from build123d import *

# Parameters (mm, degrees)
F2_R     = 1.575
F3_DEPTH = 4
F4_COUNT = 2
F5_R     = 5
F6_R     = 2.5
F7_R     = 0.5
F8_SIZE  = 1
F9_SIZE  = 0.25


with BuildPart() as f1:
    # F0 (on Right) → F1 (revolve)
    with BuildSketch(Plane.YZ):
        with BuildLine():
            Line((16.36, 0), (14, 0))
            Line((14, 0), (14, -4))
            Line((14, -4), (18, -4))
            Line((18, -4), (18, -1.64))
            ThreePointArc((18, -1.64), (16.8403448789, -1.1596551211), (16.36, 0))
        make_face()
    revolve(axis=Axis((0, 0, -0.7442336064), (0, 0, -1)))

    # F2 (on face) → F3 (join, through all)
    with BuildSketch(Plane.XY):
        with BuildLine():
            Line((-8.1, 2.5), (-9.9233440343, 2.5))
            ThreePointArc((-9.9233440343, 2.5), (-10.7587622743, 3.003635948), (-11.7060032895, 3.2366751357))
            ThreePointArc((-11.7060032895, 3.2366751357), (-12.8521864455, 3.9515520359), (-12.95875, 5.2981882222))
            ThreePointArc((-12.95875, 5.2981882222), (-14, 0), (-12.95875, -5.2981882222))
            ThreePointArc((-12.95875, -5.2981882222), (-12.8521864455, -3.9515520359), (-11.7060032895, -3.2366751357))
            ThreePointArc((-11.7060032895, -3.2366751357), (-10.7587622743, -3.003635948), (-9.9233440343, -2.5))
            Line((-9.9233440343, -2.5), (-8.1, -2.5))
            Line((-8.1, -2.5), (-8.1, -5))
            Line((-8.1, -5), (-6.6, -5))
            Line((-6.6, -5), (-4.1, -2.5))
            Line((-4.1, -2.5), (-4.1, 2.5))
            Line((-4.1, 2.5), (-6.6, 5))
            Line((-6.6, 5), (-8.1, 5))
            Line((-8.1, 5), (-8.1, 2.5))
        make_face()
        with Locations((-12, 0)):
            Circle(F2_R, mode=Mode.SUBTRACT)
    extrude(amount=-F3_DEPTH)

    # F4: F1 ×2 about axis
    f4_axis = Axis((0, 0, 0), (0, 0, -1))


with BuildPart() as f1_1:
    add(f1.part)
    for i in range(1, F4_COUNT):
        add(f1.part.rotate(f4_axis, i * 360 / F4_COUNT))

    # F5
    f5_edges = [f1_1.edges().sort_by_distance(p)[0] for p in [
        (-4.1, -2.5, -2),
        (-4.1, 2.5, -2),
        (4.1, 2.5, -2),
        (4.1, -2.5, -2),
    ]]
    fillet(f5_edges, radius=F5_R)

    # F6
    f6_edges = [f1_1.edges().sort_by_distance(p)[0] for p in [
        (-9.923344, 2.5, -2),
        (-9.923344, -2.5, -2),
        (9.923344, 2.5, -2),
        (9.923344, -2.5, -2),
    ]]
    fillet(f6_edges, radius=F6_R)

    # F7
    f7_edges = [f1_1.edges().sort_by_distance(p)[0] for p in [
        (-8.1, 2.5, -2),
        (-8.1, -2.5, -2),
        (8.1, -2.5, -2),
        (8.1, 2.5, -2),
    ]]
    fillet(f7_edges, radius=F7_R)

    # F8
    f8_edges = [f1_1.edges().sort_by_distance(p)[0] for p in [
        (0, -18, -4),
    ]]
    chamfer(f8_edges, length=F8_SIZE)

    # F9
    f9_edges = [f1_1.edges().sort_by_distance(p)[0] for p in [
        (13.575, 0, -4),
        (-13.575, 0, -4),
    ]]
    chamfer(f9_edges, length=F9_SIZE)


solid = f1_1.part
Check sheet for the modelled part. Datum: model origin and axes. Units: mm. Give positions to 0.01 mm unless a question says otherwise; leave off trailing zeros. Order: outer loops, then holes, each group sorted by start corner. A loop starts at its lowest first (then second) coordinate and runs counter-clockwise, first axis right, second up. Notation, with made-up numbers: M 59,-13 L 71,-13 A15 cw 71,8 Z; hole C -9.5,-17 d4. An arc over 180 degrees is marked long. Answer as CSV lines item,"result". Start each with the question number.
Item 1: Cross-section at A-A on x = 0. Enter the section's corners in (y, z), plus the area to 3 significant figures.
Item 2: Cross-section at C-C on z = -2.5. State how many separate pieces and enclosed holes the cut face has, plus the area to 3 significant figures.
Item 3: Thickness scan on line 1 (X direction, y = -4, z = -3.3); line 2 (Y direction, x = 12, z = -1.75) (3 decimals); line 3 (X direction, y = 3.5, z = -3). Record the ranges inside material, lowest first. Write a range as [from, to].
Item 4: Gauge pin test, flat ends, axial feed: P1, Ø1.6, axis at y = -4, z = -1.5, coming from the -X side; P2, Ø0.6, axis at x = 9, z = -1.5, coming from the -Y side; P3, Ø4, axis at x = -12, y = 0, coming from the -Z side; P4, Ø2, axis at x = -10, z = -1.5, coming from the +Y side. Record the tip position at first contact, or that the pin passes through.
Item 5: Cross-section at B-B on y = 0. Enter the section's corners in (x, z) (3 decimals).
Item 6: Mould release check, pull along Y, two halves, no side actions. Record for faces 1 (the face through (-4.47, 2.32, -2.03)), 2 (the face through (17.847, -2.343, -2.31)), 3 (the face through (4.49, 2.37, -2.03)): +Y half, -Y half, draft (parallel to the pull), parting line (faces both ways), or undercut.
Established:
1,outline,"M -18,-3 L -17,-4 L -14,-4 L -14,0 L -16.36,0 A1.64 cw -18,-1.64 Z; M 14,-4 L 17,-4 L 18,-3 L 18,-1.64 A1.64 cw 16.36,0 L 14,0 Z"
1,area,"26.8 mm^2"
2,separate pieces,"1"
2,enclosed holes,"3"
2,area,"524 mm^2"
3,line 1,"x = [-17.24, -12.88], [-8.1, -5.6], [5.6, 8.1], [12.88, 17.24]"
3,line 2,"y = [-13.416, -7.211], [-3.293, -1.575], [1.575, 3.293], [7.211, 13.416]"
3,line 3,"x = [-17.66, -12.43], [-8.1, -5.15], [5.15, 8.1], [12.43, 17.66]"
4,P1,"stops at x = -17.71"
4,P2,"stops at y = -15.74"
4,P3,"stops at z = -4"
4,P4,"stops at y = 15.58"
5,outline,"M -18,-3 L -17,-4 L -13.825,-4 L -13.575,-3.75 L -13.575,0 L -16.36,0 A1.64 cw -18,-1.64 Z; M -10.425,-3.75 L -10.175,-4 L -4.1,-4 L -4.1,0 L -10.425,0 Z; M 4.1,-4 L 10.175,-4 L 10.425,-3.75 L 10.425,0 L 4.1,0 Z; M 13.575,-3.75 L 13.825,-4 L 17,-4 L 18,-3 L 18,-1.64 A1.64 cw 16.36,0 L 13.575,0 Z"
6,face 1,"undercut"
6,face 2,"parting line"
6,face 3,"undercut"
